Autodesk Fusion 360 part; units mm, degrees
sketch "Sketch1" plane through (0, 0, 0) normal (0, 1, 0) x (1, 0, 0)
  line L0 (0, 0) -> (15.875, 0)
  line L1 (15.875, 0) -> (15.875, -88.9)
  line L2 (15.875, -88.9) -> (0, -88.9)
  line L3 (0, -88.9) -> (0, 0)
  line L4 (0, -88.9) -> (15.875, -88.9)
  line L5 (15.875, -88.9) -> (15.875, -82.55)
  line L6 (15.875, -82.55) -> (0, -82.55)
  line L7 (0, -82.55) -> (0, -88.9)
  line L8 (0, -82.55) -> (15.875, -82.55)
  line L9 (15.875, -82.55) -> (15.875, -50.8)
  line L10 (15.875, -50.8) -> (0, -50.8)
  line L11 (0, -50.8) -> (0, -82.55)
  line L12 (0, -50.8) -> (15.875, -50.8)
  line L13 (15.875, -50.8) -> (15.875, -38.1)
  line L14 (15.875, -38.1) -> (0, -38.1)
  line L15 (0, -38.1) -> (0, -50.8)
  line L16 (0, -38.1) -> (15.875, -38.1)
  line L17 (15.875, -38.1) -> (15.875, -6.35)
  line L18 (15.875, -6.35) -> (0, -6.35)
  line L19 (0, -6.35) -> (0, -38.1)
  line L20 (15.875, -88.9) -> (18.875, -88.9)
  line L21 (18.875, -88.9) -> (18.875, 0)
  line L22 (18.875, 0) -> (15.875, 0)
  line L23 (15.875, 0) -> (15.875, -88.9)
  line L24 (15.875, -88.9) -> (7.1438, -88.9)
  line L25 (7.1438, -88.9) -> (7.1438, 0)
  line L26 (7.1438, 0) -> (15.875, 0)
  line L27 (15.875, 0) -> (15.875, -88.9)
  circle A0 centre (7.1438, -82.55) radius 3.125
  circle A1 centre (7.1438, -50.8) radius 3.125
  circle A2 centre (7.1438, -38.1) radius 3.125
  circle A3 centre (7.1438, -6.35) radius 3.125
  dimension "d1" = 15.875
  dimension "d2" = 88.9
  dimension "d3" = 6.35
  dimension "d4" = 31.75
  dimension "d5" = 12.7
  dimension "d6" = 31.75
  dimension "d7" = 3
  dimension "d8" = 8.7312
  dimension "d9" = 6.25
  dimension "d10" = 6.25
  dimension "d11" = 6.25
  dimension "d12" = 6.25
extrude "Extrude1" add sketch "Sketch1" along normal blind 3 contours L0 L3 L18 L25 A3 | L0 L1 L18 L23 L25 L26 L27 A3 | L3 L14 L16 L18 L19 L25 A2 A3 | L3 L10 L12 L14 L15 L16 L25 A1 A2 | L1 L14 L16 L17 L18 L23 L25 L27 A2 A3 | L3 L6 L8 L10 L11 L12 L25 A0 A1 | L1 L10 L12 L13 L14 L16 L23 L25 L27 A1 A2 | L2 L3 L4 L6 L7 L8 L25 A0 | L1 L6 L8 L9 L10 L12 L23 L25 L27 A0 A1 | L1 L2 L4 L5 L6 L8 L23 L24 L25 L27 A0
fillet "Fillet1" radius 3 1 edges at (0, 1.5, 88.9)
fillet "Fillet2" radius 3 1 edges at (0, 1.5, 0)
extrude "Extrude2" add 1 faces at (15.875, 2, 29.6333) along direction (1, 0, 0) blind 160
sketch "Sketch2" plane through (0, 0, 0) normal (0, -1, 0) x (1, 0, 0)
  circle A0 centre (7.1438, 38.1) radius 3.125
  circle A1 centre (7.1438, 50.8) radius 3.125
  circle A2 centre (7.1438, 82.55) radius 3.125
  circle A3 centre (7.1438, 6.35) radius 3.125
  arc A4 (0, 3) -> (3, 0) centre (3, 3) ccw
  line L0 (3, 0) -> (175.875, 0)
  line L1 (175.875, 0) -> (175.875, 88.9)
  line L2 (175.875, 88.9) -> (3, 88.9)
  arc A5 (3, 88.9) -> (0, 85.9) centre (3, 85.9) ccw
  line L3 (0, 85.9) -> (0, 3)
  line L4 (175.875, 88.9) -> (165.875, 88.9)
  line L5 (165.875, 88.9) -> (165.875, 0)
  line L6 (165.875, 0) -> (175.875, 0)
  line L7 (175.875, 0) -> (175.875, 88.9)
  line L8 (165.875, 88.9) -> (145.875, 88.9)
  line L9 (145.875, 88.9) -> (145.875, 0)
  line L10 (145.875, 0) -> (165.875, 0)
  line L11 (165.875, 0) -> (165.875, 88.9)
  line L12 (145.875, 88.9) -> (135.875, 88.9)
  line L13 (135.875, 88.9) -> (135.875, 0)
  line L14 (135.875, 0) -> (145.875, 0)
  line L15 (145.875, 0) -> (145.875, 88.9)
  line L16 (135.875, 88.9) -> (115.875, 88.9)
  line L17 (115.875, 88.9) -> (115.875, 0)
  line L18 (115.875, 0) -> (135.875, 0)
  line L19 (135.875, 0) -> (135.875, 88.9)
  line L20 (115.875, 88.9) -> (105.875, 88.9)
  line L21 (105.875, 88.9) -> (105.875, 0)
  line L22 (105.875, 0) -> (115.875, 0)
  line L23 (115.875, 0) -> (115.875, 88.9)
  line L24 (105.875, 88.9) -> (85.875, 88.9)
  line L25 (85.875, 88.9) -> (85.875, 0)
  line L26 (85.875, 0) -> (105.875, 0)
  line L27 (105.875, 0) -> (105.875, 88.9)
  line L28 (85.875, 88.9) -> (75.875, 88.9)
  line L29 (75.875, 88.9) -> (75.875, 0)
  line L30 (75.875, 0) -> (85.875, 0)
  line L31 (85.875, 0) -> (85.875, 88.9)
  line L32 (75.875, 88.9) -> (55.875, 88.9)
  line L33 (55.875, 88.9) -> (55.875, 0)
  line L34 (55.875, 0) -> (75.875, 0)
  line L35 (75.875, 0) -> (75.875, 88.9)
  line L36 (55.875, 88.9) -> (45.875, 88.9)
  line L37 (45.875, 88.9) -> (45.875, 0)
  line L38 (45.875, 0) -> (55.875, 0)
  line L39 (55.875, 0) -> (55.875, 88.9)
  line L40 (45.875, 88.9) -> (25.875, 88.9)
  line L41 (25.875, 88.9) -> (25.875, 0)
  line L42 (25.875, 0) -> (45.875, 0)
  line L43 (45.875, 0) -> (45.875, 88.9)
  line L44 (25.875, 88.9) -> (15.875, 88.9)
  line L45 (15.875, 88.9) -> (15.875, 0)
  line L46 (15.875, 0) -> (25.875, 0)
  line L47 (25.875, 0) -> (25.875, 88.9)
  line L48 (15.875, 0) -> (175.875, 0)
  line L49 (175.875, 0) -> (175.875, 44.45)
  line L50 (175.875, 44.45) -> (15.875, 44.45)
  line L51 (15.875, 44.45) -> (15.875, 0)
  line L52 (145.875, 44.45) -> (165.875, 44.45)
  line L53 (165.875, 44.45) -> (165.875, 76.45)
  line L54 (165.875, 76.45) -> (145.875, 76.45)
  line L55 (145.875, 76.45) -> (145.875, 44.45)
  line L56 (145.875, 44.45) -> (165.875, 44.45)
  line L57 (165.875, 44.45) -> (165.875, 12.45)
  line L58 (165.875, 12.45) -> (145.875, 12.45)
  line L59 (145.875, 12.45) -> (145.875, 44.45)
  line L60 (115.875, 44.45) -> (135.875, 44.45)
  line L61 (135.875, 44.45) -> (135.875, 76.45)
  line L62 (135.875, 76.45) -> (115.875, 76.45)
  line L63 (115.875, 76.45) -> (115.875, 44.45)
  line L64 (115.875, 44.45) -> (135.875, 44.45)
  line L65 (135.875, 44.45) -> (135.875, 12.45)
  line L66 (135.875, 12.45) -> (115.875, 12.45)
  line L67 (115.875, 12.45) -> (115.875, 44.45)
  line L68 (85.875, 44.45) -> (105.875, 44.45)
  line L69 (105.875, 44.45) -> (105.875, 76.45)
  line L70 (105.875, 76.45) -> (85.875, 76.45)
  line L71 (85.875, 76.45) -> (85.875, 44.45)
  line L72 (85.875, 44.45) -> (105.875, 44.45)
  line L73 (105.875, 44.45) -> (105.875, 12.45)
  line L74 (105.875, 12.45) -> (85.875, 12.45)
  line L75 (85.875, 12.45) -> (85.875, 44.45)
  line L76 (55.875, 44.45) -> (75.875, 44.45)
  line L77 (75.875, 44.45) -> (75.875, 76.45)
  line L78 (75.875, 76.45) -> (55.875, 76.45)
  line L79 (55.875, 76.45) -> (55.875, 44.45)
  line L80 (55.875, 44.45) -> (75.875, 44.45)
  line L81 (75.875, 44.45) -> (75.875, 12.45)
  line L82 (75.875, 12.45) -> (55.875, 12.45)
  line L83 (55.875, 12.45) -> (55.875, 44.45)
  line L84 (25.875, 44.45) -> (45.875, 44.45)
  line L85 (45.875, 44.45) -> (45.875, 76.45)
  line L86 (45.875, 76.45) -> (25.875, 76.45)
  line L87 (25.875, 76.45) -> (25.875, 44.45)
  line L88 (25.875, 44.45) -> (45.875, 44.45)
  line L89 (45.875, 44.45) -> (45.875, 12.45)
  line L90 (45.875, 12.45) -> (25.875, 12.45)
  line L91 (25.875, 12.45) -> (25.875, 44.45)
  dimension "d21" = 10
  dimension "d22" = 20
  dimension "d23" = 10
  dimension "d24" = 20
  dimension "d25" = 10
  dimension "d26" = 20
  dimension "d27" = 10
  dimension "d28" = 20
  dimension "d29" = 10
  dimension "d30" = 20
  dimension "d31" = 10
  dimension "d32" = 32
  dimension "d33" = 32
  dimension "d34" = 32
  dimension "d35" = 32
  dimension "d36" = 32
  dimension "d37" = 32
  dimension "d38" = 32
  dimension "d39" = 32
  dimension "d40" = 32
  dimension "d41" = 32
extrude "Extrude3" cut sketch "Sketch2" against normal blind 3 contours L37 L41 L43 L47 L50 L84 L88 L89 L90 L91 | L37 L41 L43 L47 L50 L84 L85 L86 L87 L88 | L29 L33 L35 L39 L50 L76 L80 L81 L82 L83 | L29 L33 L35 L39 L50 L76 L77 L78 L79 L80 | L21 L25 L27 L31 L50 L68 L72 L73 L74 L75 | L21 L25 L27 L31 L50 L68 L69 L70 L71 L72 | L13 L17 L19 L23 L50 L60 L64 L65 L66 L67 | L13 L17 L19 L23 L50 L60 L61 L62 L63 L64 | L5 L9 L11 L15 L50 L52 L56 L57 L58 L59 | L5 L9 L11 L15 L50 L52 L53 L54 L55 L56
sketch "Sketch3" plane through (0, 0, 0) normal (0, -1, 0) x (1, 0, 0)
  line L0 (85.875, 76.45) -> (105.875, 76.45)
  line L1 (105.875, 76.45) -> (105.875, 12.45)
  line L2 (105.875, 12.45) -> (85.875, 12.45)
  line L3 (85.875, 12.45) -> (85.875, 76.45)
  line L4 (55.875, 76.45) -> (75.875, 76.45)
  line L5 (75.875, 76.45) -> (75.875, 12.45)
  line L6 (75.875, 12.45) -> (55.875, 12.45)
  line L7 (55.875, 12.45) -> (55.875, 76.45)
  line L8 (115.875, 76.45) -> (135.875, 76.45)
  line L9 (135.875, 76.45) -> (135.875, 12.45)
  line L10 (135.875, 12.45) -> (115.875, 12.45)
  line L11 (115.875, 12.45) -> (115.875, 76.45)
  line L12 (25.875, 76.45) -> (45.875, 76.45)
  line L13 (45.875, 76.45) -> (45.875, 12.45)
  line L14 (45.875, 12.45) -> (25.875, 12.45)
  line L15 (25.875, 12.45) -> (25.875, 76.45)
  line L16 (145.875, 76.45) -> (165.875, 76.45)
  line L17 (165.875, 76.45) -> (165.875, 12.45)
  line L18 (165.875, 12.45) -> (145.875, 12.45)
  line L19 (145.875, 12.45) -> (145.875, 76.45)
  circle A0 centre (7.1438, 38.1) radius 3.125
  circle A1 centre (7.1438, 50.8) radius 3.125
  circle A2 centre (7.1438, 82.55) radius 3.125
  circle A3 centre (7.1438, 6.35) radius 3.125
  arc A4 (0, 3) -> (3, 0) centre (3, 3) ccw
  line L20 (3, 0) -> (175.875, 0)
  line L21 (175.875, 0) -> (175.875, 88.9)
  line L22 (175.875, 88.9) -> (3, 88.9)
  arc A5 (3, 88.9) -> (0, 85.9) centre (3, 85.9) ccw
  line L23 (0, 85.9) -> (0, 3)
  line L24 (175.875, 88.9) -> (155.875, 88.9)
  line L25 (155.875, 88.9) -> (155.875, 0)
  line L26 (155.875, 0) -> (175.875, 0)
  line L27 (175.875, 0) -> (175.875, 88.9)
  line L28 (155.875, 88.9) -> (125.875, 88.9)
  line L29 (125.875, 88.9) -> (125.875, 0)
  line L30 (125.875, 0) -> (155.875, 0)
  line L31 (155.875, 0) -> (155.875, 88.9)
  line L32 (125.875, 88.9) -> (95.875, 88.9)
  line L33 (95.875, 88.9) -> (95.875, 0)
  line L34 (95.875, 0) -> (125.875, 0)
  line L35 (125.875, 0) -> (125.875, 88.9)
  line L36 (95.875, 88.9) -> (65.875, 88.9)
  line L37 (65.875, 88.9) -> (65.875, 0)
  line L38 (65.875, 0) -> (95.875, 0)
  line L39 (95.875, 0) -> (95.875, 88.9)
  line L40 (65.875, 88.9) -> (35.875, 88.9)
  line L41 (35.875, 88.9) -> (35.875, 0)
  line L42 (35.875, 0) -> (65.875, 0)
  line L43 (65.875, 0) -> (65.875, 88.9)
  line L44 (175.875, 88.9) -> (35.875, 88.9)
  line L45 (35.875, 88.9) -> (35.875, 82.675)
  line L46 (35.875, 82.675) -> (175.875, 82.675)
  line L47 (175.875, 82.675) -> (175.875, 88.9)
  line L48 (175.875, 0) -> (35.875, 0)
  line L49 (35.875, 0) -> (35.875, 6.225)
  line L50 (35.875, 6.225) -> (175.875, 6.225)
  line L51 (175.875, 6.225) -> (175.875, 0)
  circle A6 centre (35.875, 82.675) radius 1.625
  circle A7 centre (65.875, 82.675) radius 1.625
  circle A8 centre (95.875, 82.675) radius 1.625
  circle A9 centre (125.875, 82.675) radius 1.625
  circle A10 centre (155.875, 82.675) radius 1.625
  circle A11 centre (35.875, 6.225) radius 1.625
  circle A12 centre (65.875, 6.225) radius 1.625
  circle A13 centre (95.875, 6.225) radius 1.625
  circle A14 centre (125.875, 6.225) radius 1.625
  circle A15 centre (155.875, 6.225) radius 1.625
  dimension "d44" = 20
  dimension "d45" = 30
  dimension "d46" = 30
  dimension "d47" = 30
  dimension "d48" = 30
  dimension "d49" = 6.225
  dimension "d50" = 6.225
  dimension "d51" = 3.25
  dimension "d52" = 3.25
  dimension "d53" = 3.25
  dimension "d54" = 3.25
  dimension "d55" = 3.25
  dimension "d56" = 3.25
  dimension "d57" = 3.25
  dimension "d58" = 3.25
  dimension "d59" = 3.25
  dimension "d60" = 3.25
extrude "Extrude4" cut sketch "Sketch3" against normal blind 3 contours L33 L39 L46 A8 | L33 L39 L46 A8 | L33 L39 L46 A8 | L33 L39 L46 A8 | L33 L39 L50 A13 | L33 L39 L50 A13 | L37 L43 L46 A7 | L37 L43 L46 A7 | L29 L35 L46 A9 | L29 L35 L46 A9 | L33 L39 L50 A13 | L33 L39 L50 A13 | L37 L43 L46 A7 | L37 L43 L46 A7 | L29 L35 L46 A9 | L29 L35 L46 A9 | L29 L35 L50 A14 | L29 L35 L50 A14 | L37 L43 L50 A12 | L37 L43 L50 A12 | L29 L35 L50 A14 | L29 L35 L50 A14 | L37 L43 L50 A12 | L37 L43 L50 A12 | L41 L46 A6 | L41 L45 L46 A6 | L25 L31 L46 A10 | L25 L31 L46 A10 | L25 L31 L46 A10 | L41 L45 A6 | L25 L31 L46 A10 | L25 L31 L50 A15 | L25 L31 L50 A15 | L41 L49 L50 A11 | L41 L50 A11 | L41 L49 A11 | L25 L31 L50 A15 | L25 L31 L50 A15
Source: CAD feature listing. Evaluate the final solid. Frame: model axes, mm. A direction names the side the tool comes from. Coordinates: 2 decimals unless noted, no trailing zeros. Loops run counter-clockwise (first coordinate to the right, second up) from the corner with the lowest first, then second, coordinate; pieces in that order, holes last. Notation, with made-up numbers: (-8, 35) -> (28, 35) arc R23 ccw to (28, 73) -> close; hole circle Ø9 at (-5, -38). An arc over 180 degrees is marked (long way). One line per item, written item: value. Start each with the question number.
Q1. Section query A-A, the plane z = 38.1. Return the cut outline in (x, y) (3 decimals).
Q2. Section query C-C, the plane z = 65. Return the cut outline in (x, y) (3 decimals), and give its area (3 significant figures).
Q3. Mould query, pull axis Z, two halves, no side actions, for faces 3 (the face through (36, 1, 12.45)), 4 (the face through (106.2, 3, 45.1)), 5 (the face through (0.86, 1.52, 88)). Classes: pulls with the +Z half, pulls with the -Z half, needs draft (parallel to the pull), parting line crosses it, or undercut.
Q4. Line query: line 1 along X through (y, z) = (1.2, 47.5) (3 decimals); line 2 along Z through (x, y) = (117, 2.1); line 3 along Z through (x, y) = (34.5, 1.8). Output: solid intervals per line, ascending.
Q5. Section query B-B, the plane x = 129.5. Return the cut outline in (y, z).
Q6. Section query D-D, the plane y = 1.75. Give the number of separate pieces and of enclosed holes in the cut face, and give its area (3 significant figures).
Q7. Set-up query: faces 1 (the face through (88, 1, 88.9)), 2 (the face through (36, 1, 76.45)). Return all of +Z, -Z, +X, -X, +Y, -Y with unobstructed straight access to the full face (end or side cutting, diameter ignored); none if empty.
Results:
1. outline: (0, 0) -> (4.019, 0) -> (4.019, 3) -> (0, 3) -> close; (10.269, 0) -> (25.875, 0) -> (25.875, 3) -> (10.269, 3) -> close; (45.875, 0) -> (55.875, 0) -> (55.875, 3) -> (45.875, 3) -> close; (75.875, 0) -> (85.875, 0) -> (85.875, 3) -> (75.875, 3) -> close; (105.875, 0) -> (115.875, 0) -> (115.875, 3) -> (105.875, 3) -> close; (135.875, 0) -> (145.875, 0) -> (145.875, 3) -> (135.875, 3) -> close; (165.875, 0) -> (175.875, 0) -> (175.875, 3) -> (165.875, 3) -> close
2. outline: (0, 0) -> (25.875, 0) -> (25.875, 3) -> (0, 3) -> close; (45.875, 0) -> (55.875, 0) -> (55.875, 3) -> (45.875, 3) -> close; (75.875, 0) -> (85.875, 0) -> (85.875, 3) -> (75.875, 3) -> close; (105.875, 0) -> (115.875, 0) -> (115.875, 3) -> (105.875, 3) -> close; (135.875, 0) -> (145.875, 0) -> (145.875, 3) -> (135.875, 3) -> close; (165.875, 0) -> (175.875, 0) -> (175.875, 3) -> (165.875, 3) -> close
2. area: 228 mm^2
3. face 3: undercut
3. face 4: needs draft
3. face 5: pulls with the +Z half
4. line 1: 0 to 25.875, 45.875 to 55.875, 75.875 to 85.875, 105.875 to 115.875, 135.875 to 145.875, 165.875 to 175.875
4. line 2: 0 to 12.45, 76.45 to 88.9
4. line 3: 0 to 5.36, 7.09 to 12.45, 76.45 to 81.81, 83.54 to 88.9
5. outline: (0, 0) -> (3, 0) -> (3, 12.45) -> (0, 12.45) -> close; (0, 76.45) -> (3, 76.45) -> (3, 88.9) -> (0, 88.9) -> close
6. separate pieces: 1
6. enclosed holes: 19
6. area: 9,030 mm^2
7. face 1: +Z, +X, -X, +Y, -Y
7. face 2: +Y, -Y
